```python
from build123d import *

# Parameters (mm, degrees)
CENTRE_HOLE_FOR_L2_DEPTH      = 40
CENTRE_HOLE_FOR_L2_DEPTH_BACK = 10
SKETCH1_R                     = 39.1
SKETCH1_R_2                   = 31.75
MAIN_STRUCTURE_DEPTH          = 60
MAIN_STRUCTURE_DEPTH_BACK     = 50
SKETCH2_W                     = 100
SKETCH2_H                     = 100
SKETCH2_R                     = 39.1
BEARING_CURVE_DEPTH           = 10
SKETCH6_R                     = 10.5
SHAFT_HOLE_DEPTH              = 10
WRIST_CUTOUT_DEPTH            = 188.082869339
SKETCH11_W                    = 25
SKETCH11_H                    = 45
SKETCH11_R                    = 2.525
BOSS_EXTRUDE1_DEPTH           = 6
SKETCH15_W                    = 19.8
SKETCH15_H                    = 7
CUT_EXTRUDE4_DEPTH            = 4
CUT_EXTRUDE5_REACH            = 190.16
CUT_EXTRUDE5_END_RADIUS       = 31.75
SKETCH16_R                    = 1.5
CUT_EXTRUDE6_DEPTH            = 168.7378908
CUT_EXTRUDE6_DEPTH_BACK       = 168.7378908
SKETCH18_R                    = 3.25
CUT_EXTRUDE7_START            = -1.5875
CUT_EXTRUDE7_DEPTH            = 1.5875
SKETCH9_R                     = 12.05
BEARING_DEPTH                 = 5
CUT_EXTRUDE8_DEPTH            = 3
SKETCH21_R                    = 3.25
SKETCH21_R_2                  = 1.65
CUT_EXTRUDE9_DEPTH            = 167.868211501
CUT_EXTRUDE10_DEPTH           = 6.35
SKETCH23_R                    = 2.275
CUT_EXTRUDE11_DEPTH           = 6
CHAMFER1_SIZE                 = 0.5
BOSS_EXTRUDE2_START           = 26
BOSS_EXTRUDE2_DEPTH           = 26


with BuildPart() as part:
    # Sketch1 → Centre Hole for L2 (new, two sides: drawn at the far end of the back side and taken through both)
    with BuildSketch(Plane.XY.offset(-CENTRE_HOLE_FOR_L2_DEPTH_BACK)):
        Circle(SKETCH1_R)
        Circle(SKETCH1_R_2, mode=Mode.SUBTRACT)
    extrude(amount=CENTRE_HOLE_FOR_L2_DEPTH + CENTRE_HOLE_FOR_L2_DEPTH_BACK)

    # Sketch2 → Main Structure (add, two sides: drawn at the far end of the back side and taken through both)
    with BuildSketch(Plane.XY.offset(40).offset(-MAIN_STRUCTURE_DEPTH_BACK)):
        Rectangle(SKETCH2_W, SKETCH2_H)
        Circle(SKETCH2_R, mode=Mode.SUBTRACT)
    extrude(amount=MAIN_STRUCTURE_DEPTH + MAIN_STRUCTURE_DEPTH_BACK)

    # Sketch3 → Bearing Curve (add)
    with BuildSketch(Plane.ZY.offset(50)):
        with BuildLine():
            Line((100, 50), (100, -50))
            ThreePointArc((100, -50), (150, 0), (100, 50))
        make_face()
    bearing_curve = extrude(amount=-BEARING_CURVE_DEPTH)

    # Upright Mirror: Bearing Curve across plane
    add(bearing_curve.mirror(Plane(origin=(0, 0, 0), x_dir=(0, 0, 1), z_dir=(1, 0, 0))))

    # Sketch6 → Shaft Hole (cut)
    with BuildSketch(Plane.ZY.offset(50)):
        with Locations((100, 0)):
            Circle(SKETCH6_R)
    extrude(amount=-SHAFT_HOLE_DEPTH, mode=Mode.SUBTRACT)

    # Sketch4 → Wrist Cutout (cut, through all)
    with BuildSketch(Plane(origin=(0, 50, 0), x_dir=(1, 0, 0), z_dir=(0, 1, 0))):
        with BuildLine():
            Line((-40, -100), (-40, -60))
            ThreePointArc((-40, -60), (-34.142135624, -45.857864376), (-20, -40))
            Line((-20, -40), (20, -40))
            ThreePointArc((20, -40), (34.142135624, -45.857864376), (40, -60))
            Line((40, -60), (40, -100))
            Line((40, -100), (-40, -100))
        make_face()
    extrude(amount=-WRIST_CUTOUT_DEPTH, mode=Mode.SUBTRACT)

    # SurfaceCut1
    split(bisect_by=Plane.ZY, keep=Keep.TOP)

    # Sketch11 → Boss-Extrude1 (add)
    with BuildSketch(Plane(origin=(0, 50, 0), x_dir=(1, 0, 0), z_dir=(0, 1, 0))):
        with Locations((-12.5, -15)):
            Rectangle(SKETCH11_W, SKETCH11_H)
        with Locations(Location((-19, 1, 0), (0, 0, 270))):
            Circle(SKETCH11_R, mode=Mode.SUBTRACT)
        with Locations(Location((-19, -31, 0), (0, 0, 270))):
            Circle(SKETCH11_R, mode=Mode.SUBTRACT)
    extrude(amount=BOSS_EXTRUDE1_DEPTH)

    # Sketch15 → Cut-Extrude4 (cut)
    with BuildSketch(Plane(origin=(0, -50, 0), x_dir=(-1, 0, 0), z_dir=(0, -1, 0))):
        with Locations((9.9, -36.5)):
            Rectangle(SKETCH15_W, SKETCH15_H)
    extrude(amount=-CUT_EXTRUDE4_DEPTH, mode=Mode.SUBTRACT)

    # Cut-Extrude5: up to this cylinder (the profile starts outside it)
    cut_extrude5_end = Plane(origin=(0, 0, 35.9), z_dir=(0, 0, 1)) * Cylinder(CUT_EXTRUDE5_END_RADIUS, 444.82, mode=Mode.PRIVATE)
    # Sketch16 → Cut-Extrude5 (cut, up to the surface)
    with BuildSketch(Plane(origin=(0, -46, 0), x_dir=(-1, 0, 0), z_dir=(0, -1, 0)), mode=Mode.PRIVATE) as cut_extrude5_sk1:
        with Locations(Location((14.65, -35.9, 0), (0, 0, 90))):
            Circle(SKETCH16_R)
    cut_extrude5_tool1 = extrude(cut_extrude5_sk1.sketch, amount=-CUT_EXTRUDE5_REACH, mode=Mode.PRIVATE) - cut_extrude5_end
    add(cut_extrude5_tool1.solids().sort_by_distance((-14.65, -46, 35.9))[0], mode=Mode.SUBTRACT)
    # Sketch16 → Cut-Extrude5 (cut, up to the surface)
    with BuildSketch(Plane(origin=(0, -46, 0), x_dir=(-1, 0, 0), z_dir=(0, -1, 0)), mode=Mode.PRIVATE) as cut_extrude5_sk2:
        with Locations(Location((5.15, -35.9, 0), (0, 0, 90))):
            Circle(SKETCH16_R)
    cut_extrude5_tool2 = extrude(cut_extrude5_sk2.sketch, amount=-CUT_EXTRUDE5_REACH, mode=Mode.PRIVATE) - cut_extrude5_end
    add(cut_extrude5_tool2.solids().sort_by_distance((-5.15, -46, 35.9))[0], mode=Mode.SUBTRACT)

    # Sketch18 → Cut-Extrude6 (cut, two sides: drawn at the far end of the back side and taken through both)
    with BuildSketch(Plane.ZY.offset(50).offset(-CUT_EXTRUDE6_DEPTH_BACK)):
        with Locations((8, 0)):
            Circle(SKETCH18_R)
        with Locations((32, 0)):
            Circle(SKETCH18_R)
    extrude(amount=CUT_EXTRUDE6_DEPTH + CUT_EXTRUDE6_DEPTH_BACK, mode=Mode.SUBTRACT)

    # Sketch19 → Cut-Extrude7 (cut)
    with BuildSketch(Plane(origin=(-40, 0, 0), x_dir=(0, 0, -1), z_dir=(1, 0, 0)).offset(CUT_EXTRUDE7_START)):
        with BuildLine():
            Line((-60, 50), (-100, 50))
            ThreePointArc((-100, 50), (-150, 0), (-100, -50))
            Line((-100, -50), (-60, -50))
            Line((-60, -50), (-60, 50))
        make_face()
    extrude(amount=CUT_EXTRUDE7_DEPTH, mode=Mode.SUBTRACT)

    # Sketch9 → Bearing (cut)
    with BuildSketch(Plane(origin=(-41.5875, 0, 0), x_dir=(0, 0, -1), z_dir=(1, 0, 0))):
        with Locations((-100, 0)):
            Circle(SKETCH9_R)
    extrude(amount=-BEARING_DEPTH, mode=Mode.SUBTRACT)

    # Sketch20 → Cut-Extrude8 (cut)
    with BuildSketch(Plane.ZY.offset(50)):
        with BuildLine():
            Line((-10, -50), (100, -50))
            ThreePointArc((100, -50), (150, 0), (100, 50))
            Line((100, 50), (-10, 50))
            Line((-10, 50), (-10, -50))
        make_face()
    extrude(amount=-CUT_EXTRUDE8_DEPTH, mode=Mode.SUBTRACT)

    # Sketch21 → Cut-Extrude9 (cut, through all)
    with BuildSketch(Plane.ZY.offset(47)):
        with Locations((3, -40)):
            Circle(SKETCH21_R)
        with Locations((27, -40)):
            Circle(SKETCH21_R)
        with Locations(Location((27, 40, 0), (0, 0, 180))):
            Circle(SKETCH21_R)
        with Locations(Location((3, 40, 0), (0, 0, 180))):
            Circle(SKETCH21_R)
        with Locations((125, 0)):
            Circle(SKETCH21_R_2)
    extrude(amount=-CUT_EXTRUDE9_DEPTH, mode=Mode.SUBTRACT)

    # Sketch22 → Cut-Extrude10 (cut)
    with BuildSketch(Plane.ZY.offset(47)):
        with BuildLine():
            Line((-10, 50), (-10, -50))
            Line((-10, -50), (100, -50))
            ThreePointArc((100, -50), (150, 0), (100, 50))
            Line((100, 50), (-10, 50))
        make_face()
    extrude(amount=-CUT_EXTRUDE10_DEPTH, mode=Mode.SUBTRACT)

    # Sketch23 → Cut-Extrude11 (cut)
    with BuildSketch(Plane(origin=(0, -50, 0), x_dir=(-1, 0, 0), z_dir=(0, -1, 0))):
        with Locations(Location((15, 3.25, 0), (0, 0, 90))):
            Circle(SKETCH23_R)
    extrude(amount=-CUT_EXTRUDE11_DEPTH, mode=Mode.SUBTRACT)

    # Chamfer1
    chamfer1_edges = [part.edges().sort_by_distance(p)[0] for p in [
        (-15, -50, -0.975),
    ]]
    chamfer(chamfer1_edges, length=CHAMFER1_SIZE)

    # Sketch24 → Boss-Extrude2 (add)
    with BuildSketch(Plane(origin=(0, 0, -10), x_dir=(-1, 0, 0), z_dir=(0, 0, -1)).offset(BOSS_EXTRUDE2_START)):
        with BuildLine():
            Line((40.65, -50), (40.65, 50))
            Line((40.65, 50), (0, 50))
            Line((0, 50), (0, 31.75))
            ThreePointArc((0, 31.75), (31.75, 0), (0, -31.75))
            Line((0, -31.75), (0, -50))
            Line((0, -50), (40.65, -50))
        make_face()
    extrude(amount=-BOSS_EXTRUDE2_DEPTH)


solid = part.part
```
Build history of the part. All positions in model axes, mm. A direction names the side the tool comes from. Coordinates: 2 decimals unless noted, no trailing zeros. Order: outer loops, then holes, each group sorted by start corner. A loop starts at its lowest first (then second) coordinate and runs counter-clockwise, first axis right, second up. Notation, with made-up numbers: M -27.5,35.5 L 9.5,35.5 A20 ccw 9.5,46.5 Z; hole C -20.5,81 d3. An arc over 180 degrees is marked long. One line per question, with ' | ' between items. Start each with the question number.
1. Mould opens along X. For faces 1 (the face through (-20, -50, 1)), 2 (the face through (-15, -44, -3)), 3 (the face through (0, -37, 1)), 4 (the face through (-16.114, -36.796, 36.225)) say: +X half, -X half, draft (parallel to the pull), parting line (faces both ways), or undercut.
2. Wall check: line 1 along Z through (x, y) = (-18, 40); line 2 along Y through (x, z) = (-38, 32); line 3 along Y through (x, z) = (-32.5, 28.5). Give the ranges that are in metal, low to high. Write a range as [from, to].
3. Cut at C-C (x = -27). Write the cut outline in (y, z) (3 decimals).
4. Flat gauge pins, fed straight in: P1, Ø5, axis at y = 40, z = 27, coming from the +X side; P2, Ø3, axis at x = -13, y = 54, coming from the +Z side; P3, Ø3.5, axis at x = -15, z = -3.25, coming from the -Y side; P4, Ø7.5, axis at x = -13, z = 37.5, coming from the -Y side. Where does each tip first touch, or does it go through?
5. Tool access for faces 5 (the face through (-12.744, -46.788, -2.954)), 6 (the face through (-39.096, 0.566, 45.372)), 7 (the face through (-19, 50, -1)), 8 (the face through (-13, 53, 37.5)), 9 (the face through (-10, -48, 33)): list every direction of +Z, -Z, +X, -X, +Y, -Y with a clear straight run to the whole face (end or side of a thin tool).
6. Cut at B-B (z = 27). Write the cut outline in (x, y).
7. Cut at D-D (x = -5.15). Write the cut outline in (y, z), plus the area to 3 significant figures.
8. Cut at A-A (y = 0). Write the cut outline in (x, z).
The answers:
1) face 1: draft | face 2: undercut | face 3: +X half | face 4: undercut
2) line 1: z = [-36, -0.25], [6.25, 23.75], [30.25, 40] | line 2: y = [-50, -3.25], [3.25, 50] | line 3: y = [-50, -42.88], [-37.12, 37.12], [42.88, 50]
3) outline: M -50,-36 L -16.705,-36 L -16.705,40 L -28.281,40 L -28.281,41.265 L -50,41.265 Z; M 16.705,-36 L 50,-36 L 50,41.265 L 28.281,41.265 L 28.281,40 L 16.705,40 Z; hole C -40,3 d6.5; hole C -40,27 d6.5; hole C 40,3 d6.5; hole C 40,27 d6.5
4) P1: passes through | P2: stops at z = 37.5 | P3: stops at y = -44 | P4: stops at y = -46
5) face 5: -Y | face 6: +Z, +X | face 7: +Y | face 8: +Z, +X, -X, +Y | face 9: +Z, +X, -Y
6) outline: M -40.65,-50 L 0,-50 L 0,-43.25 L -40.65,-43.25 Z; M -40.65,-36.75 L 0,-36.75 L 0,-31.75 A31.75 cw 0,31.75 L 0,36.75 L -40.65,36.75 Z; M -40.65,43.25 L 0,43.25 L 0,56 L -25,56 L -25,50 L -40.65,50 Z
7) outline: M -50,-36 L -31.33,-36 L -31.33,34.4 L -46,34.4 L -46,33 L -50,33 Z; M -46,37.4 L -31.33,37.4 L -31.33,40 L -46,40 Z; M 31.33,-36 L 50,-36 L 50,-7.5 L 56,-7.5 L 56,37.5 L 50,37.5 L 50,40 L 31.33,40 Z; hole C -40,3 d6.5; hole C -40,27 d6.5; hole C 40,3 d6.5; hole C 40,27 d6.5 | area: 2,900 mm2
8) outline: M -40.65,-36 L -31.75,-36 L -31.75,4.75 L -40.65,4.75 Z; M -40.65,11.25 L -31.75,11.25 L -31.75,28.75 L -40.65,28.75 Z; M -40.65,35.25 L -31.75,35.25 L -31.75,40 L -39.1,40 L -39.1,54.07 A20 cw -40,60 L -40.65,60 Z
